Input: part model. Units: mm. Frame: model coordinates. Coordinates: 2 decimals unless noted, no trailing zeros. Use one line per item in the form item = value. Start each with the question number.
1) Pin query (flat end, axial travel): pin 1 (0.5 mm diameter, centred on y = -5, z = 78.5, fed in from +X); pin 2 (3 mm diameter, centred on x = 0, z = 479.5, fed in from +Y); pin 3 (8.5 mm diameter, centred on x = 0, z = -300, fed in from +Y); pin 4 (0.5 mm diameter, centred on y = -5, z = -176.5, fed in from -X). Return the tip coordinate at first contact, or that it passes through.
2) Ray query, line 1 along X through (y, z) = (0, 243); line 2 along X through (y, z) = (-0.5, 120); line 3 along Y through (x, z) = (-3.25, 239.5). Return the intervals inside material, ascending.
3) Section query A-A on x = 0. Count the separate pieces of the cut face and the enclosed holes in it, then the cut area to 3 significant figures.
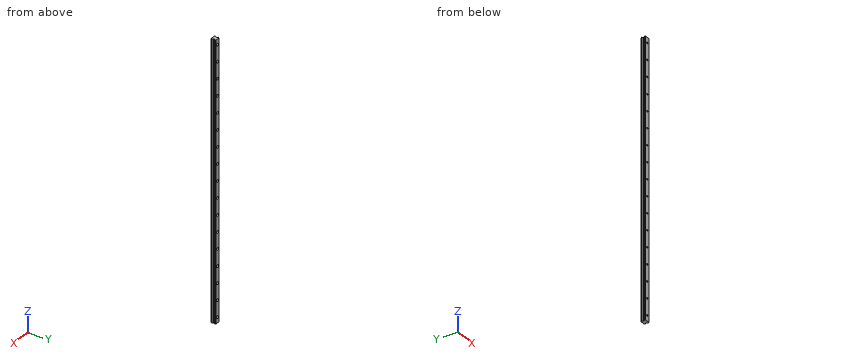
from build123d import *

# Parameters (mm, degrees)
BODY_DEPTH                     = 500
CBORE_FOR_M6_SHCS1_D           = 6
CBORE_FOR_M6_SHCS1_CBORE_D     = 9.5
CBORE_FOR_M6_SHCS1_CBORE_DEPTH = 8.4
LP_CBORE_COUNT                 = 17
LP_CBORE_PITCH                 = 60


with BuildPart() as part:
    # Sketch10 → BODY (new, symmetric)
    with BuildSketch(Plane.XY):
        with BuildLine():
            Line((-10, -10.338492954), (-10, -13))
            Line((-10, -13), (-9, -14))
            Line((-9, -14), (9, -14))
            Line((9, -14), (10, -13))
            Line((10, -13), (10, -10.338492954))
            ThreePointArc((10, -10.338492954), (9.92387953, -9.955809511), (9.707106773, -9.631386153))
            Line((9.707106773, -9.631386153), (6.892893227, -6.817172607))
            ThreePointArc((6.892893227, -6.817172607), (6.67612047, -6.492749249), (6.6, -6.110065806))
            Line((6.6, -6.110065806), (6.6, -4.549934184))
            ThreePointArc((6.6, -4.549934184), (6.67612047, -4.167250741), (6.892893227, -3.842827383))
            Line((6.892893227, -3.842827383), (7.63016236, -3.10555825))
            ThreePointArc((7.63016236, -3.10555825), (7.773916138, -2.959214094), (7.846806387, -2.767462244))
            ThreePointArc((7.846806387, -2.767462244), (8.396388302, -1.732072251), (9.431778289, -1.182490324))
            ThreePointArc((9.431778289, -1.182490324), (9.571491852, -1.133183296), (9.69062239, -1.045098237))
            Line((9.69062239, -1.045098237), (9.85355341, -0.8821672))
            ThreePointArc((9.85355341, -0.8821672), (9.961939771, -0.719955532), (10, -0.528613829))
            Line((10, -0.528613829), (10, 0.528613829))
            ThreePointArc((10, 0.528613829), (9.961939771, 0.719955532), (9.85355341, 0.8821672))
            Line((9.85355341, 0.8821672), (9.69062239, 1.045098237))
            ThreePointArc((9.69062239, 1.045098237), (9.568212026, 1.140675286), (9.422379794, 1.194081559))
            ThreePointArc((9.422379794, 1.194081559), (8.396063845, 1.741777544), (7.848162084, 2.767983654))
            ThreePointArc((7.848162084, 2.767983654), (7.775191194, 2.958001328), (7.63253117, 3.10318943))
            Line((7.63253117, 3.10318943), (7.2357206, 3.5))
            Line((7.2357206, 3.5), (-7.2357206, 3.5))
            Line((-7.2357206, 3.5), (-7.63253117, 3.10318943))
            ThreePointArc((-7.63253117, 3.10318943), (-7.775191194, 2.958001328), (-7.848162084, 2.767983654))
            ThreePointArc((-7.848162084, 2.767983654), (-8.396063845, 1.741777544), (-9.422379794, 1.194081559))
            ThreePointArc((-9.422379794, 1.194081559), (-9.568212026, 1.140675286), (-9.69062239, 1.045098237))
            Line((-9.69062239, 1.045098237), (-9.85355341, 0.8821672))
            ThreePointArc((-9.85355341, 0.8821672), (-9.961939771, 0.719955532), (-10, 0.528613829))
            Line((-10, 0.528613829), (-10, -0.528613829))
            ThreePointArc((-10, -0.528613829), (-9.961939771, -0.719955532), (-9.85355341, -0.8821672))
            Line((-9.85355341, -0.8821672), (-9.69062239, -1.045098237))
            ThreePointArc((-9.69062239, -1.045098237), (-9.571491852, -1.133183296), (-9.431778289, -1.182490324))
            ThreePointArc((-9.431778289, -1.182490324), (-8.396388302, -1.732072251), (-7.846806387, -2.767462244))
            ThreePointArc((-7.846806387, -2.767462244), (-7.773916138, -2.959214094), (-7.63016236, -3.10555825))
            Line((-7.63016236, -3.10555825), (-6.892893227, -3.842827383))
            ThreePointArc((-6.892893227, -3.842827383), (-6.67612047, -4.167250741), (-6.6, -4.549934184))
            Line((-6.6, -4.549934184), (-6.6, -6.110065806))
            ThreePointArc((-6.6, -6.110065806), (-6.67612047, -6.492749249), (-6.892893227, -6.817172607))
            Line((-6.892893227, -6.817172607), (-9.707106773, -9.631386153))
            ThreePointArc((-9.707106773, -9.631386153), (-9.92387953, -9.955809511), (-10, -10.338492954))
        make_face()
    extrude(amount=BODY_DEPTH, both=True)

    # CBORE for M6 SHCS1 (through all)
    with Locations(Plane(origin=(0, 3.5, 0), x_dir=(1, 0, 0), z_dir=(0, 1, 0))):
        with Locations((0, -480)):
            cbore_for_m6_shcs1 = CounterBoreHole(CBORE_FOR_M6_SHCS1_D / 2, CBORE_FOR_M6_SHCS1_CBORE_D / 2, CBORE_FOR_M6_SHCS1_CBORE_DEPTH)

    # MIRROR FIRST COUNTERBORE: CBORE for M6 SHCS1 across plane
    add(cbore_for_m6_shcs1.mirror(Plane.XY), mode=Mode.SUBTRACT)

    # LP CBORE: CBORE for M6 SHCS1 ×17
    with Locations(*[(0, 0, -i * LP_CBORE_PITCH) for i in range(1, LP_CBORE_COUNT)]):
        add(cbore_for_m6_shcs1, mode=Mode.SUBTRACT)


solid = part.part
Answers below:
q1.pin_1 = 6.6
q1.pin_2 = through
q1.pin_3 = -4.9
q1.pin_4 = -6.6
q2.line_1 = -10 to -3.68, 3.68 to 10
q2.line_2 = -10 to -4.75, 4.75 to 10
q2.line_3 = -14 to -4.9
q3.separate_pieces = 18
q3.enclosed_holes = 0
q3.area = 15,200 mm^2
